Source: CAD feature listing. Evaluate the final solid. Frame: model axes, mm. A direction names the side the tool comes from. Coordinates: 2 decimals unless noted, no trailing zeros. Write each loop counter-clockwise with the first axis right and the second up, starting at its lowest first coordinate (ties: lowest second). Pieces come first, ordered by that corner, then holes. Notation, with made-up numbers: (-4, -18) - (17, -18) arc R19 ccw to (17, -13) - close; hole circle Ø9 at (71, 17.25). An arc over 180 degrees is marked (long way). One line per question, with ' | ' between items. Start each with the question number.
Q1. Cut plane A-A, the plane x = 47.5. Return loops of the section in (y, z).
Q2. Cut plane B-B, the plane y = -15. Return loops of the section in (x, z), plus the area to 3 significant figures.
Q3. Cut plane D-D, the plane y = -5.75. Return loops of the section in (x, z).
Q4. Cut plane C-C, the plane z = -0.75. Return loops of the section in (x, y), plus the area to 3 significant figures.
Q5. Line query: line 1 (X direction, y = -15.5, z = 11); line 2 (Y direction, x = -1.5, z = 3); line 3 (X direction, y = -10.75, z = 3.75). Output: solid intervals per line, ascending.
Q6. Contact query for a flat-ended pin moving along its axis: P1, Ø5, axis at x = 2, z = 3.5, coming from the +Y side. Output: stop coordinate, or through.
Q7. Draft query along Y for faces 1 (the face through (13, -15, 12.81)), 2 (the face through (21, -30, 5)), 3 (the face through (46, -5, 5)). Return one class per face: +Y half, -Y half, draft (parallel to the pull), parting line (faces both ways), or undercut.
Q8. Access query for faces 4 (the face through (59.09, -15, 5)), 5 (the face through (9.09, -15, 5)). Directions: +Z, -Z, +X, -X, +Y, -Y. A direction counts if a zero-diameter tool reaches every point of the face in a straight line with its end or side. Return the directions, or none.
```python
from build123d import *

# Parameters (mm, degrees)
F0_W     = 75
F0_H     = 15
F1_DEPTH = 30
F2_W     = 20
F2_H     = 20
F3_DEPTH = 15
F4_R     = 10
F5_DEPTH = 15
F6_W     = 15
F6_H     = 20
F7_DEPTH = 15


with BuildPart() as f1:
    # F0 (on Front) → F1 (new body)
    with BuildSketch(Plane.XZ):
        with Locations((21.590133, 5.310398)):
            Rectangle(F0_W, F0_H)
    extrude(amount=F1_DEPTH)

    # F2 (on face) → F3 (cut)
    with BuildSketch(Plane.XY.offset(12.810398)):
        with Locations((-0.909867, -15)):
            Rectangle(F2_W, F2_H)
    extrude(amount=-F3_DEPTH, mode=Mode.SUBTRACT)

    # F4 (on face) → F5 (cut)
    with BuildSketch(Plane.XY.offset(12.810398)):
        with Locations((24.090133, -15)):
            Circle(F4_R)
    extrude(amount=-F5_DEPTH, mode=Mode.SUBTRACT)

    # F6 (on face) → F7 (cut)
    with BuildSketch(Plane.XY.offset(12.810398)):
        with Locations((46.590133, -15)):
            Rectangle(F6_W, F6_H)
    extrude(amount=-F7_DEPTH, mode=Mode.SUBTRACT)


solid = f1.part
```
Reply:
1) outline: (-30, -2.19) - (-25, -2.19) - (-25, 12.81) - (-30, 12.81) - close; (-5, -2.19) - (0, -2.19) - (0, 12.81) - (-5, 12.81) - close
2) outline: (-15.91, -2.19) - (-10.91, -2.19) - (-10.91, 12.81) - (-15.91, 12.81) - close; (9.09, -2.19) - (14.09, -2.19) - (14.09, 12.81) - (9.09, 12.81) - close; (34.09, -2.19) - (39.09, -2.19) - (39.09, 12.81) - (34.09, 12.81) - close; (54.09, -2.19) - (59.09, -2.19) - (59.09, 12.81) - (54.09, 12.81) - close | area: 300 mm^2
3) outline: (-15.91, -2.19) - (-10.91, -2.19) - (-10.91, 12.81) - (-15.91, 12.81) - close; (9.09, -2.19) - (20.29, -2.19) - (20.29, 12.81) - (9.09, 12.81) - close; (27.89, -2.19) - (39.09, -2.19) - (39.09, 12.81) - (27.89, 12.81) - close; (54.09, -2.19) - (59.09, -2.19) - (59.09, 12.81) - (54.09, 12.81) - close
4) outline: (-15.91, -30) - (59.09, -30) - (59.09, 0) - (-15.91, 0) - close; hole (-10.91, -25) - (9.09, -25) - (9.09, -5) - (-10.91, -5) - close; hole circle Ø20 at (24.09, -15); hole (39.09, -25) - (54.09, -25) - (54.09, -5) - (39.09, -5) - close | area: 1,240 mm^2
5) line 1: x = -15.91 to -10.91, 9.09 to 14.1, 34.08 to 39.09, 54.09 to 59.09 | line 2: y = -30 to -25, -5 to 0 | line 3: x = -15.91 to -10.91, 9.09 to 15.04, 33.14 to 39.09, 54.09 to 59.09
6) P1: stops at y = 0
7) face 1: draft | face 2: -Y half | face 3: undercut
8) face 4: +Z, -Z, +X, +Y, -Y | face 5: +Z, -Z
